Check sheet for the modelled part. Datum: model origin and axes. Units: mm. A direction names the side the tool comes from. Give positions to 0.01 mm unless a question says otherwise; leave off trailing zeros. Loops run counter-clockwise (first coordinate to the right, second up) from the corner with the lowest first, then second, coordinate; pieces in that order, holes last. Notation, with made-up numbers: (-20.5, 80) - (0.5, 80) arc R26 cw to (0.5, 114) - close; hole circle Ø3 at (35.5, 27). An arc over 180 degrees is marked (long way). Use CSV: the item, a comma, the result in double quotes.
from build123d import *

# Parameters (mm, degrees)
F1_DEPTH = 25
F0_W     = 10
F0_H     = 7.5
F2_DEPTH = 10
F3_DEPTH = 3.125
F5_R     = 2.5
F6_R     = 6.3817313598
F7_DEPTH = 30.0010045886
F7_TAPER = 10
F8_R     = 2.5


with BuildPart() as f1:
    # F0 (on Front) → F1 (new body, symmetric)
    with BuildSketch(Plane.XZ):
        Polygon((16.25, -3.75), (16.25, 3.75), (8.75, 3.75), (-16.25, 3.75), (-16.25, -3.75), align=None)
    extrude(amount=F1_DEPTH, both=True)

    # F0 (on Front) → F2 (join, symmetric)
    with BuildSketch(Plane.XZ):
        with BuildLine():
            Line((8.75, 3.75), (16.25, 3.75))
            Line((16.25, 3.75), (16.25, 10.63))
            ThreePointArc((16.25, 10.63), (18.0805826176, 15.0494173824), (22.5, 16.88))
            Line((22.5, 16.88), (23.75, 16.88))
            Line((23.75, 16.88), (23.75, 24.38))
            Line((23.75, 24.38), (22.5, 24.38))
            add(Edge.make_bspline(
                [(21.641459386, 24.3531704797), (21.9284637446, 24.3648296115), (22.2146783802, 24.37378971), (22.5, 24.38)],
                knots=[43.1879789216, 43.1879789216, 43.1879789216, 43.1879789216, 43.8994236864, 43.8994236864, 43.8994236864, 43.8994236864], degree=3))
            ThreePointArc((21.641459386, 24.3531704797), (12.4783376269, 20.0442861269), (8.75, 10.63))
            Line((8.75, 10.63), (8.75, 3.75))
        make_face()
        with Locations((28.75, 20.63)):
            Rectangle(F0_W, F0_H)
    extrude(amount=F2_DEPTH, both=True)

    # F0 (on Front) → F3 (join, symmetric)
    with BuildSketch(Plane.XZ):
        with BuildLine():
            Line((-16.25, 3.75), (8.75, 3.75))
            Line((8.75, 3.75), (8.75, 10.63))
            ThreePointArc((8.75, 10.63), (12.4783376269, 20.0442861269), (21.641459386, 24.3531704797))
            add(Edge.make_bspline(
                [(-16.25, 3.75), (-16.1136864782, 12.9915711447), (4.2189709464, 23.645407395), (21.641459386, 24.3531704797)],
                knots=[0, 0, 0, 0, 43.1879789216, 43.1879789216, 43.1879789216, 43.1879789216], degree=3))
        make_face()
    extrude(amount=F3_DEPTH, both=True)

    # F0 (on Front) → F4 (revolve)
    with BuildSketch(Plane.XZ):
        Polygon((33.75, 24.38), (33.75, 16.88), (33.75, 15.0000045886), (43.75, 15.0000045886), (43.75, 26.2500045886), (33.75, 26.2500045886), align=None)
    revolve(axis=Axis((33.75, 0, 20.6250045886), (0, 0, 1)))

    # F5
    f5_edges = [f1.edges().sort_by_distance(p)[0] for p in [
        (16.25, -25, 0),
        (-16.25, -25, 0),
        (-16.25, 25, 0),
        (16.25, 25, 0),
    ]]
    fillet(f5_edges, radius=F5_R)

    # F6 (on face) → F7 (cut, through all)
    with BuildSketch(Plane.XY.offset(26.2500045886)):
        with Locations((33.75, 0)):
            Circle(F6_R)
    extrude(amount=-F7_DEPTH, taper=F7_TAPER, mode=Mode.SUBTRACT)

    # F8
    f8_edges = [f1.edges().sort_by_distance(p)[0] for p in [
        (27.368269, 0, 26.250005),
        (29.351947, 0, 15.000005),
    ]]
    fillet(f8_edges, radius=F8_R)


solid = f1.part
1. Go/stop test with flat-tipped pins: pin 1 Ø10 at (y, z) = (6.5, 17.5) entering from +X; pin 2 Ø7.5 at (y, z) = (-5.5, 8.5) entering from -X; pin 3 Ø10 at (y, z) = (2, 10) entering from -X. Record where each tip stops, or that it passes through.
Completed:
pin 1,"stops at x = 43.64"
pin 2,"stops at x = -15.96"
pin 3,"stops at x = -16.11"
2. Sectioned sample at B-B, the plane y = 13.5. Record the boundary of the cut face in (x, z), and give its area (3 significant figures).
Completed:
outline,"(-16.25, -3.75) - (16.25, -3.75) - (16.25, 3.75) - (-16.25, 3.75) - close"
area,"244 mm²"
3. Sectioned sample at A-A, the plane z = 3. Record the boundary of the cut face in (x, y), and give its area (3 significant figures).
Completed:
outline,"(-16.25, -22.5) arc R2.5 ccw to (-13.75, -25) - (13.75, -25) arc R2.5 ccw to (16.25, -22.5) - (16.25, 22.5) arc R2.5 ccw to (13.75, 25) - (-13.75, 25) arc R2.5 ccw to (-16.25, 22.5) - close"
area,"1,620 mm²"
4. Set-up check for faces 1 (the face through (8.75, 7, 7)), 2 (the face through (38, -7, 15)), 3 (the face through (12.58, -6.61, 20.15)): record each of +Z, -Z, +X, -X, +Y, -Y from which the full face is reachable in a straight line by a thin tool's end or side.
Completed:
face 1,"+Z, -X, +Y"
face 2,"-Z, +X, +Y, -Y"
face 3,"+Z, -X, -Y"
5. Scan lines: line 1 along Y through (x, z) = (-1, 14) (3 decimals); line 2 along Z through (x, y) = (-7.5, 15); line 3 along X through (y, z) = (-4.5, 11). Record each from-to range of solid material in increasing order.
Completed:
line 1,"y = -3.125 to 3.125"
line 2,"z = -3.75 to 3.75"
line 3,"x = 8.75 to 16.26"
6. Release check for a two-part mould opening along X. For faces 4 (the face through (38.68, -2.04, 20.32)), 5 (the face through (23.5, 0.7, 16.88)), 6 (the face through (15.537, 24.248, 0.053)), 7 (the face through (23.6, -0.8, 24.38)) record: released by +X, released by -X, zero draft, split by the parting line, or undercut.
Completed:
face 4,"undercut"
face 5,"undercut"
face 6,"released by +X"
face 7,"zero draft"
